Geometry: see drawing. Coordinates: mm, zero at the bounding-box minimum. Give positions to 0.01 mm unless a question says otherwise; leave off trailing zeros. Loops run counter-clockwise (first coordinate to the right, second up) from the corner with the lowest first, then second, coordinate; pieces in that order, holes last. Notation, with made-up numbers: (44, 10) - (56, 10) arc R27 ccw to (56, 32) - close; hole circle Ø10 at (76.5, 81). An arc over 180 degrees is marked (long way). Use one line per item in the form item = value.
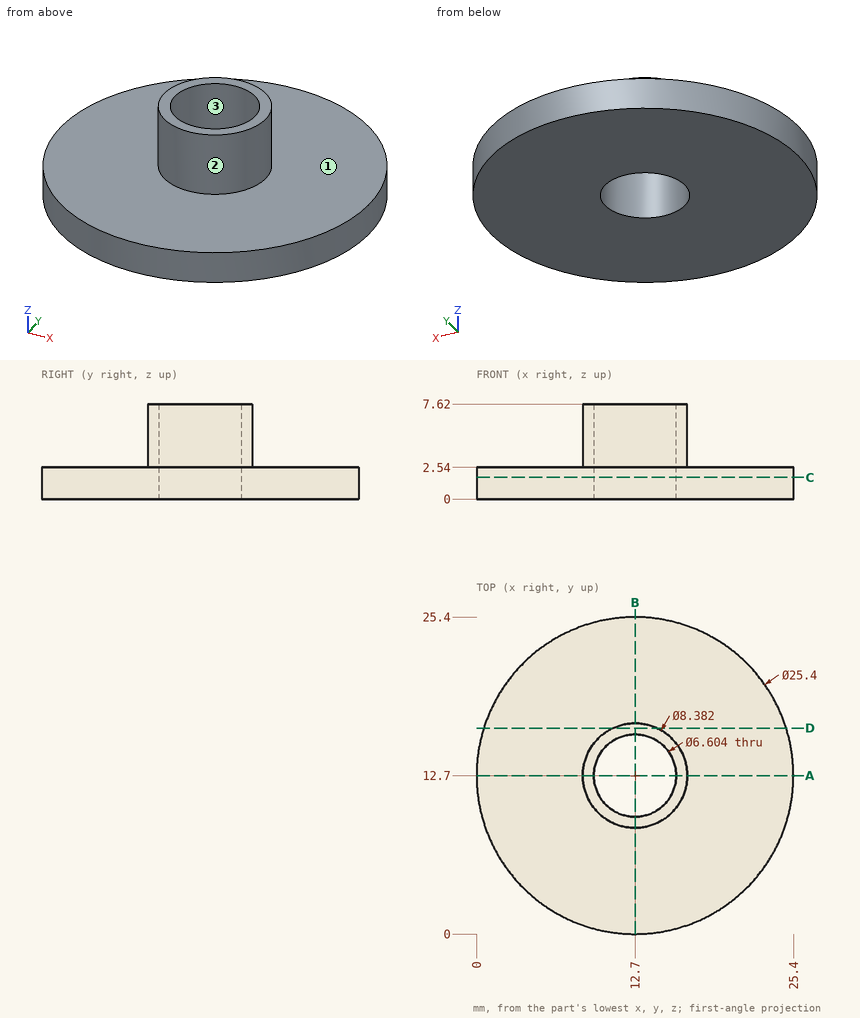
(1) Pin query (flat end, axial travel): P1, Ø4, axis at y = 5, z = 3.5, coming from the +X side; P2, Ø3, axis at x = 14, z = 3, coming from the -Y side; P3, Ø1.5, axis at x = 3, y = 13.5, coming from the +Z side; P4, Ø1, axis at y = 21.5, z = 2.5, coming from the +X side. Return the tip coordinate at first contact, or that it passes through.
Solution:
P1 = 23.92
P2 = 0
P3 = 2.54
P4 = 22.31
(2) Cut plane C-C (z = 1.75). Return the cut outline in (x, y), plus the area to 3 significant figures.
Solution:
outline = circle Ø25.4 at (12.7, 12.7); hole circle Ø6.6 at (12.7, 12.7)
area = 472 mm2
(3) Pull-direction query (Y, two-part tool) for the marked faces 1, 2 and 3; classes: released by +Y, released by -Y, zero draft, split by the parting line, or undercut.
Solution:
face_1 = zero draft
face_2 = split by the parting line
face_3 = undercut
(4) Cut plane A-A (y = 12.7). Return the cut outline in (x, z), plus the area to 3 significant figures.
Solution:
outline = (0, 0) - (9.4, 0) - (9.4, 7.62) - (8.51, 7.62) - (8.51, 2.54) - (0, 2.54) - close; (16, 0) - (25.4, 0) - (25.4, 2.54) - (16.89, 2.54) - (16.89, 7.62) - (16, 7.62) - close
area = 56.8 mm2
(5) Material intervals for L1, parallel to Y at x = 12.7, z = 2.75; L2, parallel to Z at x = 5.25, y = 15, sorted ascending. Write a range as from..to.
Solution:
L1 = 8.51..9.4, 16..16.89
L2 = 0..2.54
(6) Cut plane D-D (y = 16.5). Return the cut outline in (x, z).
Solution:
outline = (0.58, 0) - (24.82, 0) - (24.82, 2.54) - (14.47, 2.54) - (14.47, 7.62) - (10.93, 7.62) - (10.93, 2.54) - (0.58, 2.54) - close
